```python
from build123d import *

# Parameters (mm, degrees)
SKETCH_3_R          = 178
EXTRUDE_3_DEPTH     = 3
SKETCH_4_R          = 10.414
SKETCH_4_R_2        = 5.3
CUT_EXTRUDE_1_DEPTH = 10
CUT_EXTRUDE_2_DEPTH = 10


with BuildPart() as part:
    # 草图3 → 凸台-拉伸3 (new body)
    with BuildSketch(Plane(origin=(0, 0, 0), x_dir=(1, 0, 0), z_dir=(0, 1, 0))):
        Circle(SKETCH_3_R)
        with BuildLine():
            Line((-25, 33.75), (-25, -67.5))
            Line((-25, -67.5), (-116.913429511, -67.5))
            ThreePointArc((-116.913429511, -67.5), (-135, 0), (-116.913429511, 67.5))
            Line((-116.913429511, 67.5), (-25, 67.5))
            Line((-25, 67.5), (-25, 33.75))
        make_face(mode=Mode.SUBTRACT)
        with BuildLine():
            Line((25, 33.75), (25, 67.5))
            Line((25, 67.5), (116.913429511, 67.5))
            ThreePointArc((116.913429511, 67.5), (135, 0), (116.913429511, -67.5))
            Line((116.913429511, -67.5), (25, -67.5))
            Line((25, -67.5), (25, 33.75))
        make_face(mode=Mode.SUBTRACT)
    extrude(amount=EXTRUDE_3_DEPTH)

    # 草图4 → 切除-拉伸1 (cut)
    with BuildSketch(Plane(origin=(0, 3, 0), x_dir=(1, 0, 0), z_dir=(0, 1, 0))):
        with Locations((115.258405333, 115.258405333)):
            Circle(SKETCH_4_R)
        with Locations((115.258405333, -115.258405333)):
            Circle(SKETCH_4_R)
        with Locations((-115.258405333, -115.258405333)):
            Circle(SKETCH_4_R)
        with Locations((-115.258405333, 115.258405333)):
            Circle(SKETCH_4_R)
        with Locations((-90.216925784, -106.480381752)):
            Circle(SKETCH_4_R_2)
        with Locations((-106.480381752, -90.216925784)):
            Circle(SKETCH_4_R_2)
        with Locations((-106.480381752, 90.216925784)):
            Circle(SKETCH_4_R_2)
        with Locations((-90.216925784, 106.480381752)):
            Circle(SKETCH_4_R_2)
        with Locations((90.216925784, 106.480381752)):
            Circle(SKETCH_4_R_2)
        with Locations((106.480381752, 90.216925784)):
            Circle(SKETCH_4_R_2)
        with Locations((106.480381752, -90.216925784)):
            Circle(SKETCH_4_R_2)
        with Locations((90.216925784, -106.480381752)):
            Circle(SKETCH_4_R_2)
    extrude(amount=-CUT_EXTRUDE_1_DEPTH, mode=Mode.SUBTRACT)

    # 草图5 → 切除-拉伸2 (cut)
    with BuildSketch(Plane(origin=(0, 3, 0), x_dir=(1, 0, 0), z_dir=(0, 1, 0))):
        with BuildLine():
            Line((95.833188406, 150), (0, 150))
            Line((0, 150), (-95.833188406, 150))
            ThreePointArc((-95.833188406, 150), (0, 178), (95.833188406, 150))
        make_face()
        with BuildLine():
            Line((150, 95.833188406), (150, 0))
            Line((150, 0), (150, -95.833188406))
            ThreePointArc((150, -95.833188406), (178, 0), (150, 95.833188406))
        make_face()
        with BuildLine():
            Line((95.833188406, -150), (0, -150))
            Line((0, -150), (-95.833188406, -150))
            ThreePointArc((-95.833188406, -150), (0, -178), (95.833188406, -150))
        make_face()
        with BuildLine():
            Line((-150, 0), (-150, -95.833188406))
            ThreePointArc((-150, -95.833188406), (-178, 0), (-150, 95.833188406))
            Line((-150, 95.833188406), (-150, 0))
        make_face()
    extrude(amount=-CUT_EXTRUDE_2_DEPTH, mode=Mode.SUBTRACT)


solid = part.part
```
The model under review builds one solid part; all positions refer to its coordinate system, in mm. A direction names the side the tool comes from. Round coordinates to 2 decimals unless told otherwise and drop trailing zeros. Loops run counter-clockwise (first coordinate to the right, second up) from the corner with the lowest first, then second, coordinate; pieces in that order, holes last. Notation, with made-up numbers: (2.25, 24.25) -> (37.25, 24.25) arc R17 cw to (37.25, 44.25) -> close; hole circle Ø7 at (-19.75, -6.75). An arc over 180 degrees is marked (long way). Answer in a Markdown table with one row per item.
1) Consider section C-C, the plane y = 1.5. Count the separate pieces of the cut face and the enclosed holes in it, plus the area to 3 significant figures.
Taken from the geometry:
| item | result |
|---|---|
| separate pieces | 1 |
| enclosed holes | 14 |
| area | 54,800 mm² |
2) Consider section A-A, the plane x = -81.5. Write out the cut boundary in (y, z).
Taken from the geometry:
| item | result |
|---|---|
| outline | (0, -150) -> (3, -150) -> (3, -67.5) -> (0, -67.5) -> close; (0, 67.5) -> (3, 67.5) -> (3, 150) -> (0, 150) -> close |
3) For pin 1 Ø8.5 at (x, z) = (106.48, 90.22) entering from +Y; pin 2 Ø1.5 at (y, z) = (2.5, -115) entering from -X, all flat-tipped, find the tip position at first contact; note any pin that passes through.
Taken from the geometry:
| item | result |
|---|---|
| pin 1 | passes through |
| pin 2 | stops at x = -136.5 |
4) Wall thickness on line 1 along Z through (x, y) = (-82.5, 2.5); line 2 along X through (y, z) = (2.85, -58); line 3 along X through (y, z) = (0.65, -56): over which ranges is each line inside the solid? List them lowest first.
Taken from the geometry:
| item | result |
|---|---|
| line 1 | z = -150 to -67.5, 67.5 to 150 |
| line 2 | x = -150 to -121.91, -25 to 25, 121.91 to 150 |
| line 3 | x = -150 to -122.84, -25 to 25, 122.84 to 150 |
5) Consider section B-B, the plane z = 32.5. Write out the cut boundary in (x, y).
Taken from the geometry:
| item | result |
|---|---|
| outline | (-150, 0) -> (-131.03, 0) -> (-131.03, 3) -> (-150, 3) -> close; (-25, 0) -> (25, 0) -> (25, 3) -> (-25, 3) -> close; (131.03, 0) -> (150, 0) -> (150, 3) -> (131.03, 3) -> close |
6) Tool access review of faces 4 (the cylindrical face through (126.25, 1.48, -125.48)), 5 (the cylindrical face through (-134.996, 1.479, 0.99)): name each direction out of +Z, -Z, +X, -X, +Y, -Y from which nothing blocks a thin tool from reaching the whole face with its end or side.
Taken from the geometry:
| item | result |
|---|---|
| face 4 | -Z, +X, +Y, -Y |
| face 5 | +Y, -Y |
7) Draft analysis for pull direction Z (two halves, no side actions). For faces 1 (the cylindrical face through (-126.25, 1.48, 125.48)), 2 (the flat face through (-2, 0, -2)), 3 (the cylindrical face through (134.996, 1.479, -0.99)), state which applies: pulls with the +Z half, pulls with the -Z half, needs draft (parallel to the pull), parting line crosses it, or undercut.
Taken from the geometry:
| item | result |
|---|---|
| face 1 | pulls with the +Z half |
| face 2 | needs draft |
| face 3 | undercut |
8) Consider section D-D, the plane z = -6. Write out the cut boundary in (x, y).
Taken from the geometry:
| item | result |
|---|---|
| outline | (-150, 0) -> (-134.87, 0) -> (-134.87, 3) -> (-150, 3) -> close; (-25, 0) -> (25, 0) -> (25, 3) -> (-25, 3) -> close; (134.87, 0) -> (150, 0) -> (150, 3) -> (134.87, 3) -> close |
